The model under review builds one solid part; all positions refer to its coordinate system, in mm. Face numbers are marked on the shaded views. A direction names the side the tool comes from. Round coordinates to 2 decimals unless told otherwise and drop trailing zeros. Write each loop counter-clockwise with the first axis right and the second up, starting at its lowest first coordinate (ties: lowest second). Pieces come first, ordered by that corner, then holes. Notation, with made-up numbers: (24.25, -29) - (56.25, -29) arc R14 ccw to (56.25, -20) - close; hole circle Ø10 at (-1.75, -19.75). An arc over 180 degrees is marked (long way). Write each question's results on one line, items separated by ' | '.
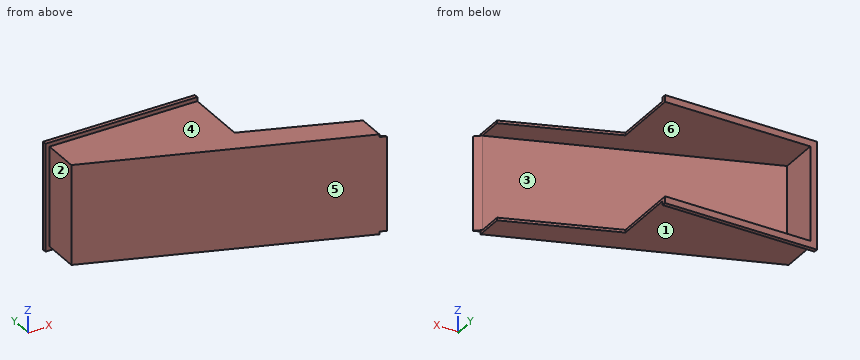
Autodesk Fusion 360 part; units mm, degrees
sketch "Sketch1" plane through (0, 0, 0) normal (0, 0, 1) x (1, 0, 0)
  line L0 (0, 0) -> (0, 30)
  line L1 (0, 0) -> (192.637, -70.1141)
  line L2 (0, 0) -> (200, 0) construction
  line L3 (192.637, -70.1141) -> (188.0053, -66.3)
  line L4 (192.637, -70.1141) -> (203.3355, -70.1141) construction
  line L5 (188.0053, -66.3) -> (2, 1.4004)
  line L6 (0, 30) -> (2, 30)
  line L7 (2, 30) -> (2, 1.4004)
  dimension "d2" = 30
  dimension "d3" = 20
  dimension "d4" = 205
  dimension "d6" = 6
  dimension "d10" = 2
  dimension "d13" = 140.529
extrude "Extrude1" add sketch "Sketch1" along normal blind 70 makes body 1
sketch "Sketch2" plane through (0, 0, 0) normal (0, 0, 1) x (1, 0, 0)
  line L0 (2, 1.4004) -> (2, 30)
  line L1 (0, 30) -> (110, 30)
  line L2 (110, 30) -> (110, -19.0179)
  line L3 (110, -19.0179) -> (188.0053, -48.1069)
  line L4 (188.0053, -66.3) -> (188.0053, -48.1069)
  line L5 (2, 30) -> (0, 30)
  line L6 (0, 30) -> (0, 0)
  line L7 (0, 30) -> (0, 29)
  line L8 (0, 0) -> (192.637, -70.1141)
  line L9 (0, 0) -> (192.7051, -70.1389)
  line L10 (188.0053, -66.3) -> (188.0053, -68.4283)
  point P0 (2, 30)
  point P1 (188.0053, -66.3)
  point P2 (0, 30)
  dimension "d16" = 110
extrude "Extrude2" add sketch "Sketch2" against normal blind 2 bodies 1
ref_plane "WorkPlane1" through (0, 0, 35) normal (0, 0, 1) x (1, 0, 0)
mirror "Mirror1" about plane through (0, 0, 35) normal (0, 0, 1) of bodies 1 makes body 2
sketch "Sketch3" plane through (0, 0, 72) normal (0, 0, 1) x (-1, 0, 0)
  line L0 (-110, -30) -> (0, -30)
  line L1 (0, -30) -> (0, 0)
  line L2 (0, 0) -> (-188.0053, 68.4283)
  line L3 (-188.0053, 68.4283) -> (-188.0053, 48.1069)
  line L4 (-188.0053, 48.1069) -> (-110, 19.0179)
  line L5 (-110, 19.0179) -> (-110, -30)
  line L6 (0, -30) -> (-110, -30)
  line L7 (-110, -30) -> (-110, -27)
  line L8 (-110, -27) -> (0, -27)
  line L9 (0, -27) -> (0, -30)
  dimension "d22" = 3
extrude "Extrude3" add sketch "Sketch3" along normal blind 3 contours L0 L1 L5 L6 L7 L8 L9 bodies 2
sketch "Sketch4" plane through (0, 0, -2) normal (0, 0, -1) x (1, 0, 0)
  line L0 (0, -30) -> (110, -30)
  line L1 (110, -30) -> (110, 19.0179)
  line L2 (110, 19.0179) -> (188.0053, 48.1069)
  line L3 (188.0053, 48.1069) -> (188.0053, 68.4283)
  line L4 (188.0053, 68.4283) -> (0, 0)
  line L5 (0, 0) -> (0, -30)
  line L6 (110, -30) -> (0, -30)
  line L7 (0, -30) -> (0, -27)
  line L8 (0, -27) -> (110, -27)
  line L9 (110, -27) -> (110, -30)
  dimension "d25" = 3
extrude "Extrude4" add sketch "Sketch4" along normal blind 3 contours L0 L1 L5 L6 L7 L8 L9 bodies 1
sketch "Sketch5" plane through (0, 0, 0) normal (-1, 0, 0) x (0, -1, 0)
  line L0 (0, 0) -> (0, 72)
  line L1 (0, 72) -> (-27, 72)
  line L2 (-27, 72) -> (-27, 75)
  line L3 (-27, 75) -> (-30, 75)
  line L4 (-30, 75) -> (-30, 0)
  line L5 (-30, 0) -> (0, 0)
  line L6 (-30, -5) -> (-27, -5)
  line L7 (-27, -5) -> (-27, 75)
  line L8 (-27, 75) -> (-30, 75)
  line L9 (-30, 75) -> (-30, -5)
  point P0 (-30, -5)
extrude "Extrude5" add sketch "Sketch5" along normal blind 3 contours L5 L6 L7 L9 | L2 L3 L4 L5 L7 L8 L9 bodies 1 2
Q1. We need section B-B (x = 145). State the section outline as (y, z) points, plus the area to 3 significant figures.
Evaluation:
outline: (-52.78, -2) - (-32.07, -2) - (-32.07, 0) - (-50.65, 0) - (-50.65, 70) - (-32.07, 70) - (-32.07, 72) - (-52.78, 72) - close | area: 232 mm^2
Q2. The part is to be moulded in two halves that separate along Z. For the marked faces 1, 2 and 3, say which applies: released by +Z, released by -Z, zero draft, split by the parting line, or undercut.
Evaluation:
face 1: released by -Z | face 2: zero draft | face 3: undercut
Q3. We need section C-C (x = 100). State the section outline as (y, z) points, plus the area to 3 significant figures.
Evaluation:
outline: (-36.4, -2) - (27, -2) - (27, -5) - (30, -5) - (30, 0) - (-34.27, 0) - (-34.27, 70) - (30, 70) - (30, 75) - (27, 75) - (27, 72) - (-36.4, 72) - close | area: 433 mm^2
Q4. We need section A-A (z = 50). State the section outline as (x, y) points, plus the area to 3 significant figures.
Evaluation:
outline: (-3, 27) - (0, 27) - (0, 0) - (192.64, -70.11) - (188.01, -66.3) - (2, 1.4) - (2, 30) - (-3, 30) - close | area: 471 mm^2
Q5. For probe 1 along Z at (x, y) = (117.5, -22.5); probe 2 along X at (y, z) = (3, 12); probe 3 along Y at (x, z) = (57.5, 67), list the stretches that pass through material, from the lowest coordinate up.
Evaluation:
probe 1: z = -2 to 0, 70 to 72 | probe 2: x = 0 to 2 | probe 3: y = -20.93 to -18.8
Q6. Tool access review of the marked faces 4, 5 and 6: name each direction out of +Z, -Z, +X, -X, +Y, -Y from which nothing blocks a thin tool from reaching the whole face with its end or side.
Evaluation:
face 4: +Z, +X, -X, -Y | face 5: +Z, -Z, -X, -Y | face 6: +X, +Y
Q7. Insertion check: P1, Ø8.5, axis at y = 18, z = 34, coming from the +X side; P2, Ø12, axis at x = 49.5, z = 37.5, coming from the -Y side; P3, Ø1, axis at y = -54, z = 71, coming from the +X side; P4, Ø8, axis at x = 93.5, y = -42.5, coming from the +Z side. Each pin has a flat end and moves straight along its axis. Give the tip position at first contact, or say it passes through.
Evaluation:
P1: stops at x = 2 | P2: stops at y = -20.2 | P3: stops at x = 188.01 | P4: passes through
